```python
from build123d import *

# Parameters (mm, degrees)
ESBO_O1_W                    = 131.4
ESBO_O1_H                    = 68.4
BASE_DEPTH                   = 1.2
FILETE1_R                    = 15
FILETE2_R                    = 15
FILETE3_R                    = 10
FILETE4_R                    = 10
PAREDES_START                = 10
PAREDES_DEPTH                = 10
FILETE_DA_BASE_R             = 3
ESBO_O6_R                    = 2.5
SUPORTE_DOS_PARAFUSOS_DEPTH  = 10
ESBO_O7_R                    = 1
FURO_PARA_OS_PARAFUSOS_DEPTH = 6
ESBO_O8_W                    = 100
ESBO_O8_H                    = 42.449361702
CORTE_EXTRUS_O1_DEPTH        = 10
ESBO_O9_W                    = 134.994270452
ESBO_O9_H                    = 14.346821692
CORTE_EXTRUS_O2_DEPTH        = 96.501256536
CHANFRO8_SIZE                = 2
CHANFRO9_SIZE                = 2
CHANFRO10_SIZE               = 2
CHANFRO11_SIZE               = 2
ESBO_O10_R                   = 1
CORTE_EXTRUS_O4_DEPTH        = 2


with BuildPart() as part:
    # Esboço1 → Base (new body)
    with BuildSketch(Plane(origin=(0, 0, 0), x_dir=(1, 0, 0), z_dir=(0, 1, 0))):
        Rectangle(ESBO_O1_W, ESBO_O1_H)
    extrude(amount=BASE_DEPTH)

    # Filete1
    filete1_edges = [part.edges().sort_by_distance(p)[0] for p in [
        (65.7, 0.6, 34.2),
    ]]
    fillet(filete1_edges, radius=FILETE1_R)

    # Filete2
    filete2_edges = [part.edges().sort_by_distance(p)[0] for p in [
        (-65.7, 0.6, 34.2),
    ]]
    fillet(filete2_edges, radius=FILETE2_R)

    # Filete3
    filete3_edges = [part.edges().sort_by_distance(p)[0] for p in [
        (65.7, 0.6, -34.2),
    ]]
    fillet(filete3_edges, radius=FILETE3_R)

    # Filete4
    filete4_edges = [part.edges().sort_by_distance(p)[0] for p in [
        (-65.7, 0.6, -34.2),
    ]]
    fillet(filete4_edges, radius=FILETE4_R)

    # Esboço5 → Paredes (add)
    with BuildSketch(Plane(origin=(0, 1.2, 0), x_dir=(1, 0, 0), z_dir=(0, 1, 0)).offset(PAREDES_START)):
        with BuildLine():
            Line((55.7, 34.2), (-55.7, 34.2))
            ThreePointArc((-55.7, 34.2), (-62.771067812, 31.271067812), (-65.7, 24.2))
            Line((-65.7, 24.2), (-65.7, -19.2))
            ThreePointArc((-65.7, -19.2), (-61.306601718, -29.806601718), (-50.7, -34.2))
            Line((-50.7, -34.2), (50.7, -34.2))
            ThreePointArc((50.7, -34.2), (61.306601718, -29.806601718), (65.7, -19.2))
            Line((65.7, -19.2), (65.7, 24.2))
            ThreePointArc((65.7, 24.2), (62.771067812, 31.271067812), (55.7, 34.2))
        make_face()
        with BuildLine():
            Line((55.7, 33), (-55.7, 33))
            ThreePointArc((-55.7, 33), (-61.922539674, 30.422539674), (-64.5, 24.2))
            Line((-64.5, 24.2), (-64.5, -19.2))
            ThreePointArc((-64.5, -19.2), (-60.45807358, -28.95807358), (-50.7, -33))
            Line((-50.7, -33), (50.7, -33))
            ThreePointArc((50.7, -33), (60.45807358, -28.95807358), (64.5, -19.2))
            Line((64.5, -19.2), (64.5, 24.2))
            ThreePointArc((64.5, 24.2), (61.922539674, 30.422539674), (55.7, 33))
        make_face(mode=Mode.SUBTRACT)
    extrude(amount=-PAREDES_DEPTH)

    # Filete da base
    filete_da_base_edges = [part.edges().sort_by_distance(p)[0] for p in [
        (65.7, 0, -2.5),
        (61.306601718, 0, 29.806601718),
        (0, 0, 34.2),
        (-61.306601718, 0, 29.806601718),
        (0, 0, -34.2),
        (62.771067812, 0, -31.271067812),
        (-65.7, 0, -2.5),
        (-62.771067812, 0, -31.271067812),
    ]]
    fillet(filete_da_base_edges, radius=FILETE_DA_BASE_R)

    # Esboço6 → Suporte dos parafusos (add)
    with BuildSketch(Plane(origin=(0, 1.2, 0), x_dir=(1, 0, 0), z_dir=(0, 1, 0))):
        with Locations(Location((-57.7, 26.2, 0), (0, 0, 90))):
            Circle(ESBO_O6_R)
        with Locations(Location((-57.7, -26.2, 0), (0, 0, 90))):
            Circle(ESBO_O6_R)
        with Locations(Location((57.7, 26.2, 0), (0, 0, 90))):
            Circle(ESBO_O6_R)
        with Locations(Location((57.7, -26.2, 0), (0, 0, 90))):
            Circle(ESBO_O6_R)
    extrude(amount=SUPORTE_DOS_PARAFUSOS_DEPTH)

    # Esboço7 → Furo para os parafusos (cut)
    with BuildSketch(Plane(origin=(0, 11.2, 0), x_dir=(1, 0, 0), z_dir=(0, 1, 0))):
        with Locations(Location((-57.7, 26.2, 0), (0, 0, 270))):
            Circle(ESBO_O7_R)
        with Locations(Location((-57.7, -26.2, 0), (0, 0, 270))):
            Circle(ESBO_O7_R)
        with Locations(Location((57.7, -26.2, 0), (0, 0, 270))):
            Circle(ESBO_O7_R)
        with Locations(Location((57.7, 26.2, 0), (0, 0, 270))):
            Circle(ESBO_O7_R)
    extrude(amount=-FURO_PARA_OS_PARAFUSOS_DEPTH, mode=Mode.SUBTRACT)

    # Esboço8 → Corte-extrusão1 (cut)
    with BuildSketch(Plane(origin=(0, 1.2, 0), x_dir=(1, 0, 0), z_dir=(0, 1, 0))):
        Rectangle(ESBO_O8_W, ESBO_O8_H)
    extrude(amount=-CORTE_EXTRUS_O1_DEPTH, mode=Mode.SUBTRACT)

    # Esboço9 → Corte-extrusão2 (cut, through all)
    with BuildSketch(Plane.XY.offset(34.2)):
        with Locations((0, 11.2)):
            Rectangle(ESBO_O9_W, ESBO_O9_H)
    extrude(amount=-CORTE_EXTRUS_O2_DEPTH, mode=Mode.SUBTRACT)

    # Chanfro8
    chanfro8_edges = [part.edges().sort_by_distance(p)[0] for p in [
        (-50, 0.6, -21.224680851),
    ]]
    chamfer(chanfro8_edges, length=CHANFRO8_SIZE)

    # Chanfro9
    chanfro9_edges = [part.edges().sort_by_distance(p)[0] for p in [
        (50, 0.6, -21.224680851),
    ]]
    chamfer(chanfro9_edges, length=CHANFRO9_SIZE)

    # Chanfro10
    chanfro10_edges = [part.edges().sort_by_distance(p)[0] for p in [
        (50, 0.6, 21.224680851),
    ]]
    chamfer(chanfro10_edges, length=CHANFRO10_SIZE)

    # Chanfro11
    chanfro11_edges = [part.edges().sort_by_distance(p)[0] for p in [
        (-50, 0.6, 21.224680851),
    ]]
    chamfer(chanfro11_edges, length=CHANFRO11_SIZE)

    # Esboço10 → Corte-extrusão4 (cut)
    with BuildSketch(Plane(origin=(0, 4.026589154, 0), x_dir=(1, 0, 0), z_dir=(0, 1, 0))):
        with Locations(Location((-57.7, 26.2, 0), (0, 0, 270))):
            Circle(ESBO_O10_R)
        with Locations(Location((-57.7, -26.2, 0), (0, 0, 270))):
            Circle(ESBO_O10_R)
    extrude(amount=-CORTE_EXTRUS_O4_DEPTH, mode=Mode.SUBTRACT)


solid = part.part
```
Can you work these out from the model? Positions are in its coordinate system, mm. A direction names the side the tool comes from. Give positions to 0.01 mm unless a question says otherwise; leave off trailing zeros. Loops run counter-clockwise (first coordinate to the right, second up) from the corner with the lowest first, then second, coordinate; pieces in that order, holes last. Notation, with made-up numbers: M 24,13.25 L 30,13.25 A10 cw 30,32.25 Z; hole C 23,-0.75 d9. An arc over 180 degrees is marked long. One line per question, with ' | ' between items. Start each with the question number.
Q1. If we mould it in two halves opening along Z, with no side actions, what happens to faces 3 (the flat face through (58, 4.027, 26)), 4 (the cylindrical face through (61.991, 2.633, -30.354)), 5 (the cylindrical face through (-61.42, 3.52, 29.69)), 6 (the cylindrical face through (-62.69, 3.52, -31.35))? For each: +Z half, -Z half, draft (parallel to the pull), parting line (faces both ways), or undercut.
Q2. If we section it at B-B (z = -0.5): Please give me the cut outline in (x, y), plus the area to 3 significant figures.
Q3. If we section it at A-A (x = -34.5): Please give me the cut outline in (y, z), plus the area to 3 significant figures.
Q4. For faces 1 (the cylindrical face through (-59.81, 2.59, 24.86)), 2 (the flat face through (-58, 4.027, 25)), which set-ups out of +Z, -Z, +X, -X, +Y, -Y let a thin tool reach every point of the face, with its end or its side?
Q5. If I drill on line 1 (Z direction, x = -20, y = 3.05); line 2 (X direction, y = 3.2, z = -26.2); line 3 (X direction, y = 3.3, z = 26.2), over which ranges is the centre line in solid material (lowest first)? Write a range as from..to.
Q6. For pin 1 Ø0.6 at (y, z) = (0.5, -6) entering from -X; pin 2 Ø1 at (y, z) = (1, 3.5) entering from +X; pin 3 Ø1 at (x, z) = (-2, -22.5) entering from +Y, each with a flat end and sliding along its axis, tell me the tip position at first contact or that it passes through.
Computed:
1) face 3: draft | face 4: undercut | face 5: +Z half | face 6: -Z half
2) outline: M -65.7,3 A3 ccw -62.7,0 L -50,0 L -50,1.2 L -64.5,1.2 L -64.5,4.03 L -65.7,4.03 Z; M 50,0 L 62.7,0 A3 ccw 65.7,3 L 65.7,4.03 L 64.5,4.03 L 64.5,1.2 L 50,1.2 Z | area: 40.6 mm²
3) outline: M 0,-31.2 A3 ccw 3,-34.2 L 4.03,-34.2 L 4.03,-33 L 1.2,-33 L 1.2,-21.22 L 0,-21.22 Z; M 0,21.22 L 1.2,21.22 L 1.2,33 L 4.03,33 L 4.03,34.2 L 3,34.2 A3 ccw 0,31.2 Z | area: 34.1 mm²
4) face 1: +Y | face 2: +Z, -Z, +X, -X, +Y
5) line 1: z = -34.2..-33, 33..34.2 | line 2: x = -65.5..-64.27, -60.2..-58.7, -56.7..-55.2, 55.2..60.2, 64.27..65.5 | line 3: x = -63.97..-62.59, -60.2..-58.7, -56.7..-55.2, 55.2..60.2, 62.59..63.97
6) pin 1: stops at x = -64.74 | pin 2: stops at x = 65.3 | pin 3: stops at y = 1.2
